from build123d import *

# Parameters (mm, degrees)
CROQUIS1_R              = 1.5
SALIENTE_EXTRUIR1_DEPTH = 3
SALIENTE_EXTRUIR2_START = 3
CROQUIS2_W              = 5
CROQUIS2_H              = 18
SALIENTE_EXTRUIR2_DEPTH = 9
REDONDEO6_R             = 9
REDONDEO7_R             = 9
CORTAR_EXTRUIR1_REACH   = 47.338
CROQUIS3_R              = 1.705559653


with BuildPart() as part:
    # Croquis1 → Saliente-Extruir1 (new body)
    with BuildSketch(Plane.XY):
        with BuildLine():
            Line((-7.68763367, 13.798076923), (22.31236633, 13.798076923))
            ThreePointArc((22.31236633, 13.798076923), (25.847900236, 12.333610829), (27.31236633, 8.798076923))
            Line((27.31236633, 8.798076923), (27.31236633, -21.201923077))
            ThreePointArc((27.31236633, -21.201923077), (25.847900236, -24.737456983), (22.31236633, -26.201923077))
            Line((22.31236633, -26.201923077), (-7.68763367, -26.201923077))
            ThreePointArc((-7.68763367, -26.201923077), (-11.223167576, -24.737456983), (-12.68763367, -21.201923077))
            Line((-12.68763367, -21.201923077), (-12.68763367, 8.798076923))
            ThreePointArc((-12.68763367, 8.798076923), (-11.223167576, 12.333610829), (-7.68763367, 13.798076923))
        make_face()
        with Locations((7.31236633, 7.298076923)):
            Circle(CROQUIS1_R, mode=Mode.SUBTRACT)
        with Locations((7.31236633, -19.701923077)):
            Circle(CROQUIS1_R, mode=Mode.SUBTRACT)
    extrude(amount=SALIENTE_EXTRUIR1_DEPTH)

    # Croquis2 → Saliente-Extruir2 (add)
    with BuildSketch(Plane.XY.offset(SALIENTE_EXTRUIR2_START)):
        with Locations((-5.18763367, -6.201923077)):
            Rectangle(CROQUIS2_W, CROQUIS2_H)
        with Locations((19.81236633, -6.201923077)):
            Rectangle(CROQUIS2_W, CROQUIS2_H)
    extrude(amount=SALIENTE_EXTRUIR2_DEPTH)

    # Redondeo6
    redondeo6_edges = [part.edges().sort_by_distance(p)[0] for p in [
        (-5.18763367, 2.798076923, 12),
        (-5.18763367, -15.201923077, 12),
    ]]
    fillet(redondeo6_edges, radius=REDONDEO6_R - 0.0001)  # a hair under: the kernel refuses the full size

    # Redondeo7
    redondeo7_edges = [part.edges().sort_by_distance(p)[0] for p in [
        (19.81236633, -15.201923077, 12),
        (19.81236633, 2.798076923, 12),
    ]]
    fillet(redondeo7_edges, radius=REDONDEO7_R - 0.0001)  # a hair under: the kernel refuses the full size

    # Cortar-Extruir1: up to this face of the body (flat: up to its plane)
    cortar_extruir1_end = Plane(part.part.faces().sort_by_distance((22.31236633, -6.201923077, 6.819731779))[0])
    # Croquis3 → Cortar-Extruir1 (cut, up to the picked face)
    with BuildSketch(Plane.ZY.offset(7.68763367), mode=Mode.PRIVATE) as cortar_extruir1_sk1:
        with Locations((7.74625312, -6.201923077)):
            Circle(CROQUIS3_R)
    cortar_extruir1_tool1 = split(extrude(cortar_extruir1_sk1.sketch, amount=-CORTAR_EXTRUIR1_REACH, mode=Mode.PRIVATE), bisect_by=cortar_extruir1_end, keep=Keep.BOTH, mode=Mode.PRIVATE)
    add(cortar_extruir1_tool1.solids().sort_by(Axis((-7.687634, -6.201923, 7.746253), (1, 0, 0)))[0], mode=Mode.SUBTRACT)


solid = part.part
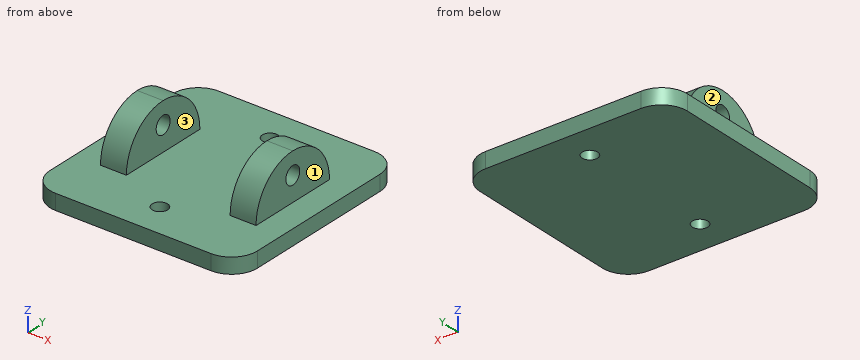
The model under review builds one solid part; all positions refer to its coordinate system, in mm. Face numbers are marked on the shaded views. A direction names the side the tool comes from. Give positions to 0.01 mm unless a question says otherwise; leave off trailing zeros. Loops run counter-clockwise (first coordinate to the right, second up) from the corner with the lowest first, then second, coordinate; pieces in that order, holes last. Notation, with made-up numbers: (9.25, 12) -> (61.25, 12) arc R19 cw to (61.25, 32) -> close; hole circle Ø4 at (37, -37). An arc over 180 degrees is marked (long way). Put each result on its own line as item: value. Start each with the question number.
1. We need section C-C on z = 8.75. State the section outline as (x, y) points, then the cut area to 3 significant figures.
2. We need section A-A on y = 8. State the section outline as (x, z) points, then the cut area to 3 significant figures.
3. Clearance check with flat-ended pins moving along their axes: P1, Ø7, axis at y = -10.5, z = 9, coming from the -X side; P2, Ø2.5, axis at y = -5, z = 8, coming from the +X side; P3, Ø6, axis at x = 16, z = 8, coming from the -Y side. State where each tip first meets the part, or that it passes through.
4. We need section D-D on z = 4.5. State the section outline as (x, y) points.
5. Wall thickness on probe 1 along Z at (x, y) = (20.5, -20); probe 2 along X at (y, z) = (-14, 3.5); probe 3 along Y at (x, z) = (-3, 3.75): over which ranges is each line inside the solid? List them lowest first.
6. For the marked faces 1, 2 and 3, list the 3-axis set-ups (+Z, -Z, +X, -X, +Y, -Y) from which the entire face can be reached by the end or side of a thin tool; tool diameter is ignored.
Determined:
1. outline: (-7.69, -13.13) -> (-2.69, -13.13) -> (-2.69, -7.58) -> (-7.69, -7.58) -> close; (-7.69, -4.82) -> (-2.69, -4.82) -> (-2.69, 0.72) -> (-7.69, 0.72) -> close; (17.31, -13.13) -> (22.31, -13.13) -> (22.31, -7.58) -> (17.31, -7.58) -> close; (17.31, -4.82) -> (22.31, -4.82) -> (22.31, 0.72) -> (17.31, 0.72) -> close
1. area: 111 mm^2
2. outline: (-12.69, 0) -> (5.99, 0) -> (5.99, 3) -> (-12.69, 3) -> close; (8.64, 0) -> (27.31, 0) -> (27.31, 3) -> (8.64, 3) -> close
2. area: 112 mm^2
3. P1: x = -7.69
3. P2: x = 22.31
3. P3: y = -14.9
4. outline: (-7.69, -15.08) -> (-2.69, -15.08) -> (-2.69, 2.67) -> (-7.69, 2.67) -> close; (17.31, -15.08) -> (22.31, -15.08) -> (22.31, 2.67) -> (17.31, 2.67) -> close
5. probe 1: 0 to 3
5. probe 2: -7.69 to -2.69, 17.31 to 22.31
5. probe 3: -15.17 to 2.77
6. face 1: +Z, +X, +Y, -Y
6. face 2: +Z, -X, +Y, -Y
6. face 3: +Z, +Y, -Y
